from build123d import *

# Parameters (mm, degrees)
F0_W      = 60
F0_H      = 55
F1_DEPTH  = 35
F2_T      = -4
F3_R      = 9.5
F3_R_2    = 8
F6_R      = 8
F7_DEPTH  = 4
F8_R      = 12.5
F8_R_2    = 11
F11_R     = 11
F12_DEPTH = 4
F13_R     = 12.5
F13_R_2   = 11
F16_DEPTH = 4


with BuildPart() as f1:
    # F0 (on Top) → F1 (new body)
    with BuildSketch(Plane.XY):
        Rectangle(F0_W, F0_H)
    extrude(amount=F1_DEPTH)

    # F2
    f2_openings = [f1.faces().sort_by_distance(p)[0] for p in [
        (0, 0, 35),
    ]]
    offset(amount=F2_T, openings=f2_openings)

    # F5: sweep along a path in F4
    with BuildLine(Plane.XZ) as f5_path:
        Line((-30, 12.8732416779), (-49.8803923108, 10.6892083519))
    # F3 (on face) → F5 (sweep)
    with BuildSketch(Plane(origin=(-30, 0, 0), x_dir=(0, -1, 0), z_dir=(-1, 0, 0))):
        with Locations((12.2240986817, 10.7874526048)):
            Circle(F3_R)
        with Locations((12.2240986817, 10.7874526048)):
            Circle(F3_R_2, mode=Mode.SUBTRACT)
    sweep(path=f5_path.line)

    # F6 (on face) → F7 (cut, through all)
    with BuildSketch(Plane(origin=(-30, 0, 0), x_dir=(0, -1, 0), z_dir=(-1, 0, 0))):
        with Locations((12.2240986817, 10.7874526048)):
            Circle(F6_R)
    extrude(amount=-F7_DEPTH, mode=Mode.SUBTRACT)

    # F10: sweep along a path in F9
    with BuildLine(Plane.XZ) as f10_path:
        Line((34.9448250159, 21.2307306323), (54.5700194764, 25.0845264738))
    # F8 (on face) → F10 (sweep)
    with BuildSketch(Plane.YZ.offset(30)):
        with Locations((-13.5, 19)):
            Circle(F8_R)
        with Locations((-13.5, 19)):
            Circle(F8_R_2, mode=Mode.SUBTRACT)
        with Locations((13.5, 19)):
            Circle(F8_R)
        with Locations((13.5, 19)):
            Circle(F8_R_2, mode=Mode.SUBTRACT)
    sweep(path=f10_path.line)

    # F11 (on face) → F12 (cut, through all)
    with BuildSketch(Plane.YZ.offset(30)):
        with Locations((13.5, 19)):
            Circle(F11_R)
        with Locations((-13.5, 19)):
            Circle(F11_R)
    extrude(amount=-F12_DEPTH, mode=Mode.SUBTRACT)

    # F15: sweep along a path in F14
    with BuildLine(Plane.YZ) as f15_path:
        Line((26.9883851239, 16.3239016038), (46.2833066753, 21.5875507492))
    # F13 (on face) → F15 (sweep)
    with BuildSketch(Plane(origin=(0, 27.5, 0), x_dir=(-1, 0, 0), z_dir=(0, 1, 0))):
        with Locations((0, 16.2113178521)):
            Circle(F13_R)
        with Locations((0, 16.2113178521)):
            Circle(F13_R_2, mode=Mode.SUBTRACT)
    sweep(path=f15_path.line)

    # F16 (cut, through all): a face of the model
    f16_faces = [f1.faces().sort_by_distance(p)[0] for p in [
        (5.559e-07, 27.5, 16.2113144868),
    ]]
    extrude(f16_faces, amount=-F16_DEPTH, mode=Mode.SUBTRACT)


solid = f1.part
Geometry: final body of the model. Coordinates: model frame, mm. A direction names the side the tool comes from. Round coordinates to 2 decimals unless told otherwise and drop trailing zeros. Loops run counter-clockwise (first coordinate to the right, second up) from the corner with the lowest first, then second, coordinate; pieces in that order, holes last. Notation, with made-up numbers: M 20.25,60.25 L 45.25,60.25 A12 ccw 45.25,64.25 Z; hole C 70.5,20 d2. An arc over 180 degrees is marked long. One line per question, with ' | ' between items.
(1) Contact query for flat-ended pins moving along their axis: P1, Ø3, axis at x = 39.5, y = 16, coming from the +Z side; P2, Ø1.5, axis at x = -17, y = -13.5, coming from the -Z side; P3, Ø3, axis at x = -37, y = -15.5, coming from the -Z side. Output: stop coordinate, or through.
Check result:
P1: stops at z = 33.5 | P2: stops at z = 0 | P3: stops at z = 0.64
(2) Material intervals for line 1 along Y through (x, z) = (29.1, 19); line 2 along Z through (x, y) = (28.1, 13.5); line 3 along Y through (x, z) = (5, 4.5), sorted ascending. Write a range as from..to.
Check result:
line 1: y = -27.5..-24.5, -2.5..2.5, 24.5..27.5 | line 2: z = 0..8, 30..35 | line 3: y = -27.5..-23.5, 23.5..27.5
(3) Pull-direction query (Y, two-part tool) for faces 4 (the flat face through (0, -24, 35)), 5 (the flat face through (0, -23.5, 19)), 6 (the flat face through (0, -27.5, 17)); classes: +Y half, -Y half, draft (parallel to the pull), parting line (faces both ways), or undercut.
Check result:
face 4: draft | face 5: undercut | face 6: -Y half
(4) Cut plane B-B on z = 25.5. Give the number of separate pieces and of enclosed holes in the cut face, plus the area to 3 significant figures.
Check result:
separate pieces: 3 | enclosed holes: 0 | area: 867 mm2
(5) Cut plane A-A on x = 17.5. Return the cut outline in (y, z), plus the area to 3 significant figures.
Check result:
outline: M -27.5,0 L 27.5,0 L 27.5,35 L 23.5,35 L 23.5,4 L -23.5,4 L -23.5,35 L -27.5,35 Z | area: 468 mm2
(6) Access query for faces 1 (the flat face through (30, 0, 17)), 2 (the flat face through (0, 0, 4)), 3 (the flat face through (-49.88, -6, 14)). Directions: +Z, -Z, +X, -X, +Y, -Y. A direction counts if a zero-diameter tool reaches every point of the face in a straight line with its end or side. Return the directions, or none.
Check result:
face 1: none | face 2: +Z | face 3: +Z, -Z, -X, +Y, -Y
